```python
from build123d import *

# Parameters (mm, degrees)
BOX003_W                = 34
BOX003_H                = 10
BOX003_DEPTH            = 6
CYLINDER006_R           = 3
CYLINDER006_DEPTH       = 34
CYLINDER006_PITCH_ANGLE = 90
BOX004_W                = 34
BOX004_H                = 6
BOX004_DEPTH            = 1
CYLINDER005_R           = 3
CYLINDER005_DEPTH       = 34
CYLINDER005_PITCH_ANGLE = 90
CYLINDER008_R           = 3
CYLINDER008_DEPTH       = 1
CYLINDER004_R           = 1.5
CYLINDER004_DEPTH       = 11
CYLINDER009_R           = 3
CYLINDER009_DEPTH       = 1
CYLINDER003_R           = 1.5
CYLINDER003_DEPTH       = 11
CYLINDER010_R           = 3
CYLINDER010_DEPTH       = 1
CYLINDER002_R           = 1.5
CYLINDER002_DEPTH       = 11
CYLINDER007_R           = 3
CYLINDER007_DEPTH       = 1
CYLINDER001_R           = 1.5
CYLINDER001_DEPTH       = 11
BOX001_W                = 22
BOX001_H                = 7
BOX001_DEPTH            = 10.2
CHAMFER_SIZE            = 2
BOX002_W                = 22
BOX002_H                = 7
BOX002_DEPTH            = 10.2
CHAMFER001_SIZE         = 2
BOX_W                   = 34
BOX_H                   = 22
BOX_DEPTH               = 10


with BuildPart() as cube003:
    # Box003 → Box003 (new body)
    with BuildSketch(Plane(origin=(0, 6, 1), x_dir=(1, 0, 0), z_dir=(0, 0, 1))):
        with Locations((17, 5)):
            Rectangle(BOX003_W, BOX003_H)
    extrude(amount=BOX003_DEPTH)


with BuildPart() as cylinder006:
    # Cylinder006 → Cylinder006 (new body)
    with BuildSketch(Plane.XY):
        Circle(CYLINDER006_R)
    extrude(amount=CYLINDER006_DEPTH)


with BuildPart() as cylinder006_1:
    # Cylinder006 pitch: moved
    add(cylinder006.part.rotate(Axis((0, 0, 0), (0, 1, 0)), CYLINDER006_PITCH_ANGLE))


with BuildPart() as cylinder006_2:
    # Cylinder006 placement: moved
    add(cylinder006_1.part.moved(Location((0, 16, 4))))


with BuildPart() as cube004:
    # Box004 → Box004 (new body)
    with BuildSketch(Plane(origin=(0, 8, 0), x_dir=(1, 0, 0), z_dir=(0, 0, 1))):
        with Locations((17, 3)):
            Rectangle(BOX004_W, BOX004_H)
    extrude(amount=BOX004_DEPTH)


with BuildPart() as fusion005:
    # Cylinder005 → Cylinder005 (new body)
    with BuildSketch(Plane.XY):
        Circle(CYLINDER005_R)
    extrude(amount=CYLINDER005_DEPTH)


with BuildPart() as fusion005_1:
    # Cylinder005 pitch: moved
    add(fusion005.part.rotate(Axis((0, 0, 0), (0, 1, 0)), CYLINDER005_PITCH_ANGLE))


with BuildPart() as fusion005_2:
    # Cylinder005 placement: moved
    add(fusion005_1.part.moved(Location((0, 6, 4))))

    # Fusion005: union Cube003, Cylinder006, Cube004
    add(cube003.part)
    add(cylinder006_2.part)
    add(cube004.part)


with BuildPart() as cylinder008:
    # Cylinder008 → Cylinder008 (new body)
    with BuildSketch(Plane(origin=(25, 1.5, 0), x_dir=(1, 0, 0), z_dir=(0, 0, 1))):
        Circle(CYLINDER008_R)
    extrude(amount=CYLINDER008_DEPTH)


with BuildPart() as fusion004:
    # Cylinder004 → Cylinder004 (new body)
    with BuildSketch(Plane(origin=(25, 1.5, 0), x_dir=(1, 0, 0), z_dir=(0, 0, 1))):
        Circle(CYLINDER004_R)
    extrude(amount=CYLINDER004_DEPTH)

    # Fusion004: union Cylinder008
    add(cylinder008.part)


with BuildPart() as fusion004_1:
    # Fusion004 placement: moved
    add(fusion004.part.moved(Location((-0.5, -0.5, 0))))


with BuildPart() as cylinder009:
    # Cylinder009 → Cylinder009 (new body)
    with BuildSketch(Plane(origin=(9, 20.5, 0), x_dir=(1, 0, 0), z_dir=(0, 0, 1))):
        Circle(CYLINDER009_R)
    extrude(amount=CYLINDER009_DEPTH)


with BuildPart() as fusion003:
    # Cylinder003 → Cylinder003 (new body)
    with BuildSketch(Plane(origin=(9, 20.5, 0), x_dir=(1, 0, 0), z_dir=(0, 0, 1))):
        Circle(CYLINDER003_R)
    extrude(amount=CYLINDER003_DEPTH)

    # Fusion003: union Cylinder009
    add(cylinder009.part)


with BuildPart() as fusion003_1:
    # Fusion003 placement: moved
    add(fusion003.part.moved(Location((0.5, 0.5, 0))))


with BuildPart() as cylinder010:
    # Cylinder010 → Cylinder010 (new body)
    with BuildSketch(Plane(origin=(25, 20.5, 0), x_dir=(1, 0, 0), z_dir=(0, 0, 1))):
        Circle(CYLINDER010_R)
    extrude(amount=CYLINDER010_DEPTH)


with BuildPart() as fusion002:
    # Cylinder002 → Cylinder002 (new body)
    with BuildSketch(Plane(origin=(25, 20.5, 0), x_dir=(1, 0, 0), z_dir=(0, 0, 1))):
        Circle(CYLINDER002_R)
    extrude(amount=CYLINDER002_DEPTH)

    # Fusion002: union Cylinder010
    add(cylinder010.part)


with BuildPart() as fusion002_1:
    # Fusion002 placement: moved
    add(fusion002.part.moved(Location((-0.5, 0.5, 0))))


with BuildPart() as cylinder007:
    # Cylinder007 → Cylinder007 (new body)
    with BuildSketch(Plane(origin=(9, 1.5, 0), x_dir=(1, 0, 0), z_dir=(0, 0, 1))):
        Circle(CYLINDER007_R)
    extrude(amount=CYLINDER007_DEPTH)


with BuildPart() as fusion001:
    # Cylinder001 → Cylinder001 (new body)
    with BuildSketch(Plane(origin=(9, 1.5, 0), x_dir=(1, 0, 0), z_dir=(0, 0, 1))):
        Circle(CYLINDER001_R)
    extrude(amount=CYLINDER001_DEPTH)

    # Fusion001: union Cylinder007
    add(cylinder007.part)


with BuildPart() as fusion001_1:
    # Fusion001 placement: moved
    add(fusion001.part.moved(Location((0.5, -0.5, 0))))


with BuildPart() as chamfer_body:
    # Box001 → Box001 (new body)
    with BuildSketch(Plane(origin=(6, -2, 0), x_dir=(1, 0, 0), z_dir=(0, 0, 1))):
        with Locations((11, 3.5)):
            Rectangle(BOX001_W, BOX001_H)
    extrude(amount=BOX001_DEPTH)

    # Chamfer
    chamfer_edges = [chamfer_body.edges().sort_by_distance(p)[0] for p in [
        (17, -2, 0),
    ]]
    chamfer(chamfer_edges, length=CHAMFER_SIZE)


with BuildPart() as chamfer001:
    # Box002 → Box002 (new body)
    with BuildSketch(Plane(origin=(6, 17, 0), x_dir=(1, 0, 0), z_dir=(0, 0, 1))):
        with Locations((11, 3.5)):
            Rectangle(BOX002_W, BOX002_H)
    extrude(amount=BOX002_DEPTH)

    # Chamfer001
    chamfer001_edges = [chamfer001.edges().sort_by_distance(p)[0] for p in [
        (17, 24, 0),
    ]]
    chamfer(chamfer001_edges, length=CHAMFER001_SIZE)


with BuildPart() as do_not_print_igus_slider:
    # Box → Box (new body)
    with BuildSketch(Plane.XY):
        with Locations((17, 11)):
            Rectangle(BOX_W, BOX_H)
    extrude(amount=BOX_DEPTH)

    # Fusion: union Chamfer body, Chamfer001
    add(chamfer_body.part)
    add(chamfer001.part)

    # Cut: cut Fusion001
    add(fusion001_1.part, mode=Mode.SUBTRACT)

    # Cut001: cut Fusion002
    add(fusion002_1.part, mode=Mode.SUBTRACT)

    # Cut002: cut Fusion003
    add(fusion003_1.part, mode=Mode.SUBTRACT)

    # Cut003: cut Fusion004
    add(fusion004_1.part, mode=Mode.SUBTRACT)

    # Cut004: cut Fusion005
    add(fusion005_2.part, mode=Mode.SUBTRACT)


solid = do_not_print_igus_slider.part
```
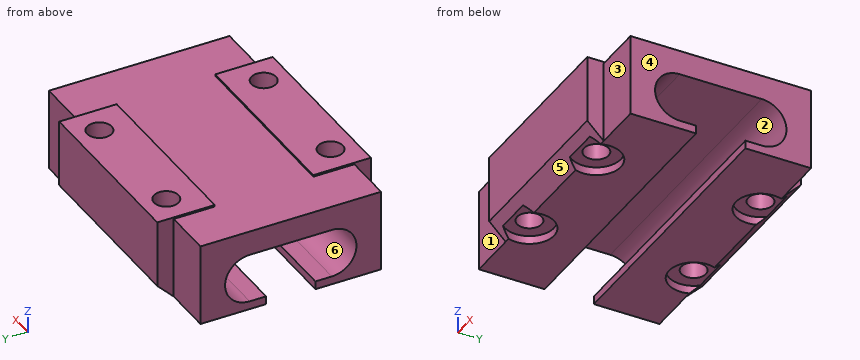
Input: part model. Units: mm. Frame: model coordinates. Face numbers are marked on the shaded views. A direction names the side the tool comes from. Round coordinates to 2 decimals unless told otherwise and drop trailing zeros. Loops run counter-clockwise (first coordinate to the right, second up) from the corner with the lowest first, then second, coordinate; pieces in that order, holes last. Notation, with made-up numbers: (55, 53.5) - (80, 53.5) arc R27 ccw to (80, 75.5) - close; hole circle Ø11 at (7.25, 15). An arc over 180 degrees is marked (long way). One line per item, written item: value. Start each with the question number.
(1) Section A-A, the plane z = 4. Return loops of the section in (x, y).
(2) Section D-D, the plane y = 21. Return loops of the section in (x, z), plus the area to 3 significant figures.
(3) Draft query along Z for the marked faces 4, 5 and 6. Return one class per face: +Z half, -Z half, draft (parallel to the pull), parting line (faces both ways), or undercut.
(4) Section C-C, the plane x = 9.5. Count the separate pieces of the cut face and the enclosed holes in it, plus the area to 3 significant figures.
(5) Access query for the marked faces 1, 2 and 3. Directions: +Z, -Z, +X, -X, +Y, -Y. A direction counts if a zero-diameter tool reaches every point of the face in a straight line with its end or side. Return the directions, or none.
(6) Section B-B, the plane z = 8.75. Return loops of the section in (x, y).
(7) Ray query, line 1 (Y direction, x = 24.5, z = 8); line 2 (X direction, y = 1, z = 0.7); line 3 (X direction, y = 21, z = 3.25). Return the intervals inside material, ascending. Write a range as [from, to].
(8) Contact query for flat-ended pins moving along their axis: P1, Ø3.5, axis at x = 24.5, y = 21, coming from the -Z side; P2, Ø0.6, axis at x = 17, y = 7, coming from the +Z side; P3, Ø0.5, axis at x = 13, z = 0.5, coming from the +Y side. Output: stop coordinate, or through.
Results below:
1. outline: (0, 0) - (6, 0) - (6, -2) - (28, -2) - (28, 0) - (34, 0) - (34, 3) - (0, 3) - close; (0, 19) - (34, 19) - (34, 22) - (28, 22) - (28, 24) - (6, 24) - (6, 22) - (0, 22) - close; hole circle Ø3 at (9.5, 1); hole circle Ø3 at (9.5, 21); hole circle Ø3 at (24.5, 1); hole circle Ø3 at (24.5, 21)
2. outline: (0, 0) - (6.5, 0) - (6.5, 1) - (8, 1) - (8, 10.2) - (6, 10.2) - (6, 10) - (0, 10) - close; (11, 1) - (12.5, 1) - (12.5, 0) - (21.5, 0) - (21.5, 1) - (23, 1) - (23, 10.2) - (11, 10.2) - close; (26, 1) - (27.5, 1) - (27.5, 0) - (34, 0) - (34, 10) - (28, 10) - (28, 10.2) - (26, 10.2) - close
2. area: 277 mm^2
3. face 4: draft
3. face 5: -Z half
3. face 6: undercut
4. separate pieces: 3
4. enclosed holes: 0
4. area: 100 mm^2
5. face 1: +Z, -Z, -X, -Y
5. face 2: +X, -X
5. face 3: +Z, -Z, +X, -Y
6. outline: (0, 0) - (6, 0) - (6, -2) - (28, -2) - (28, 0) - (34, 0) - (34, 22) - (28, 22) - (28, 24) - (6, 24) - (6, 22) - (0, 22) - close; hole circle Ø3 at (9.5, 1); hole circle Ø3 at (9.5, 21); hole circle Ø3 at (24.5, 1); hole circle Ø3 at (24.5, 21)
7. line 1: [-2, -0.5], [2.5, 19.5], [22.5, 24]
7. line 2: [0, 6.5], [12.5, 21.5], [27.5, 34]
7. line 3: [0, 8], [11, 23], [26, 34]
8. P1: z = 1
8. P2: z = 10
8. P3: y = 22.75
